For this review, take the finished solid that the model builds, in its own axes (mm). A direction names the side the tool comes from. Round coordinates to 2 decimals unless told otherwise and drop trailing zeros. Write each loop counter-clockwise with the first axis right and the second up, starting at its lowest first coordinate (ties: lowest second). Pieces come first, ordered by that corner, then holes.
from build123d import *

# Parameters (mm, degrees)
F2_T = -2.5
F3_R = 8


with BuildPart() as f1:
    # F0 (on Front) → F1 (revolve)
    with BuildSketch(Plane.XZ):
        Polygon((0, 243), (0, 0), (36, 0), (36, 189.3837451935), (23, 200), (23, 240), (26.3027578132, 240), (26.3027578132, 243), align=None)
    revolve(axis=Axis((0, 0, 121.5), (0, 0, 1)))

    # F2
    f2_openings = [f1.faces().sort_by_distance(p)[0] for p in [
        (0, 0, 243),
    ]]
    offset(amount=F2_T, openings=f2_openings, kind=Kind.INTERSECTION)

    # F3
    f3_edges = [f1.edges().sort_by_distance(p)[0] for p in [
        (-36, 0, 0),
        (-36, 0, 189.383745),
    ]]
    fillet(f3_edges, radius=F3_R)


solid = f1.part
(1) For line 1 along Y through (x, z) = (0, 91.5); line 2 along Y through (x, z) = (0, 242); line 3 along Z through (x, y) = (3, -4), list the stretches that pass through material, from the lowest coordinate up.
Geometry check:
line 1: y = -36 to -33.5, 33.5 to 36
line 2: y = -26.3 to -20.5, 20.5 to 26.3
line 3: z = 0 to 2.5
(2) Mouldability with a two-part tool opening along Y and no side actions: class faces 4 (the face through (-4.444, -20.013, 220.963)), 5 (the face through (34.34, 10.81, 98.04)), 6 (the face through (0, 0, 0)) as pulls with the +Y half, pulls with the -Y half, needs draft (parallel to the pull), parting line crosses it, or undercut.
Geometry check:
face 4: undercut
face 5: parting line crosses it
face 6: needs draft
(3) For faces 1 (the face through (-5.16, -23.237, 242.754)), 2 (the face through (10.84, -20.84, 199.6)), 3 (the face through (-20, -14, 243)), list the 3-axis set-ups (+Z, -Z, +X, -X, +Y, -Y) from which the entire face can be reached by the end or side of a thin tool; tool diameter is ignored.
Geometry check:
face 1: +Z
face 2: none
face 3: +Z, +X, -X, +Y, -Y
(4) We need section A-A, the plane z = 141. Give the boundary of the cut face in (x, y), and give its area (3 significant figures).
Geometry check:
outline: circle Ø72 at (0, 0); hole circle Ø67 at (0, 0)
area: 546 mm2
(5) For pin 1 Ø8 at (x, z) = (2.5, 101) entering from +Y; pin 2 Ø1 at (y, z) = (27, 31) entering from -X; pin 3 Ø4 at (x, y) = (-14.5, 14.5) entering from +Z; pin 4 Ø2 at (x, z) = (-26.5, 117.5) entering from +Y, all flat-tipped, find the tip position at first contact; note any pin that passes through.
Geometry check:
pin 1: stops at y = 36
pin 2: stops at x = -24.37
pin 3: stops at z = 242.5
pin 4: stops at y = 25.41
